```python
from build123d import *

# Parameters (mm, degrees)
SKETCH1_R               = 1.6
BOSS_EXTRUDE1_DEPTH     = 2
SKETCH2_W               = 12
SKETCH2_H               = 12
BOSS_EXTRUDE2_DEPTH     = 6
CUT_EXTRUDE1_DEPTH      = 4
CUT_EXTRUDE1_DEPTH_BACK = 25.093567606
SKETCH2_3_W             = 8
SKETCH2_3_H             = 10
FILLET1_R               = 4
FILLET3_R               = 1
CHAMFER1_SIZE           = 1


with BuildPart() as part:
    # Sketch1 → Boss-Extrude1 (new body)
    with BuildSketch(Plane.XY):
        with BuildLine():
            Line((-12.5, -16.5), (12.5, -16.5))
            ThreePointArc((12.5, -16.5), (15.328427125, -15.328427125), (16.5, -12.5))
            Line((16.5, -12.5), (16.5, 12.5))
            ThreePointArc((16.5, 12.5), (15.328427125, 15.328427125), (12.5, 16.5))
            Line((12.5, 16.5), (-12.5, 16.5))
            ThreePointArc((-12.5, 16.5), (-15.328427125, 15.328427125), (-16.5, 12.5))
            Line((-16.5, 12.5), (-16.5, -12.5))
            ThreePointArc((-16.5, -12.5), (-15.328427125, -15.328427125), (-12.5, -16.5))
        make_face()
        with Locations((-12.5, -12.5)):
            Circle(SKETCH1_R, mode=Mode.SUBTRACT)
        with Locations((12.5, -12.5)):
            Circle(SKETCH1_R, mode=Mode.SUBTRACT)
        with Locations((12.5, 12.5)):
            Circle(SKETCH1_R, mode=Mode.SUBTRACT)
        with Locations((-12.5, 12.5)):
            Circle(SKETCH1_R, mode=Mode.SUBTRACT)
    extrude(amount=BOSS_EXTRUDE1_DEPTH)

    # Sketch2 → Boss-Extrude2 (add)
    with BuildSketch(Plane.XY.offset(2)):
        with Locations((0, -10.5)):
            Rectangle(SKETCH2_W, SKETCH2_H)
    extrude(amount=BOSS_EXTRUDE2_DEPTH)

    # Sketch2<3> → Cut-Extrude1 (cut, two sides: drawn at the far end of the back side and taken through both)
    with BuildSketch(Plane.XY.offset(2).offset(-CUT_EXTRUDE1_DEPTH_BACK)):
        with Locations((0, -11.5)):
            Rectangle(SKETCH2_3_W, SKETCH2_3_H)
    extrude(amount=CUT_EXTRUDE1_DEPTH + CUT_EXTRUDE1_DEPTH_BACK, mode=Mode.SUBTRACT)

    # Fillet1
    fillet1_edges = [part.edges().sort_by_distance(p)[0] for p in [
        (0, -4.5, 8),
    ]]
    fillet(fillet1_edges, radius=FILLET1_R)

    # Fillet3
    fillet3_edges = [part.edges().sort_by_distance(p)[0] for p in [
        (-6, -12.5, 8),
        (-6, -10.5, 2),
        (0, -4.5, 2),
        (6, -10.5, 2),
        (-6, -4.5, 3),
        (6, -4.5, 3),
        (6, -12.5, 8),
        (6, -5.671572875, 6.828427125),
        (-6, -5.671572875, 6.828427125),
    ]]
    fillet(fillet3_edges, radius=FILLET3_R)

    # Chamfer1
    chamfer1_edges = [part.edges().sort_by_distance(p)[0] for p in [
        (-15.328427125, -15.328427125, 2),
        (-9.75, -16.5, 2),
        (15.328427125, -15.328427125, 2),
        (16.5, 0, 2),
        (15.328427125, 15.328427125, 2),
        (0, 16.5, 2),
        (-15.328427125, 15.328427125, 2),
        (-6, -16.5, 5),
        (0, -16.5, 8),
        (9.75, -16.5, 2),
        (6, -16.5, 5),
        (5.707106781, -16.5, 7.707106781),
        (-5.707106781, -16.5, 7.707106781),
        (-16.5, 0, 2),
        (-6.292893219, -16.5, 2.292893219),
        (6.292893219, -16.5, 2.292893219),
    ]]
    chamfer(chamfer1_edges, length=CHAMFER1_SIZE)


solid = part.part
```
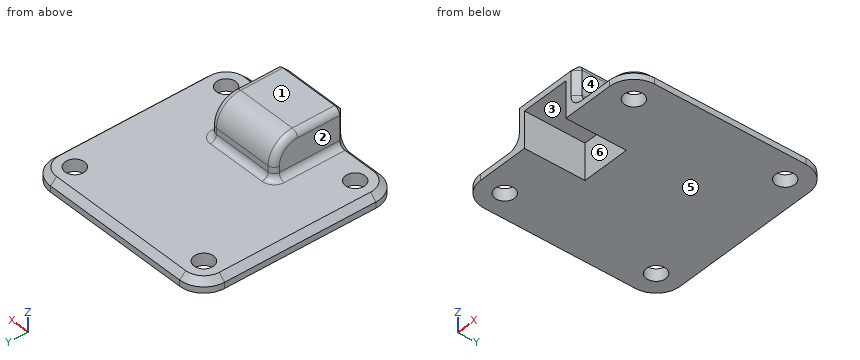
For this review, take the finished solid that the model builds, in its own axes (mm). Face numbers are marked on the shaded views. A direction names the side the tool comes from. Give positions to 0.01 mm unless a question says otherwise; leave off trailing zeros. Write each loop counter-clockwise with the first axis right and the second up, starting at its lowest first coordinate (ties: lowest second). Pieces come first, ordered by that corner, then holes.
Item 1: Take a section at A-A (x = -2). Give the boundary of the cut face in (y, z).
Item 2: The part is to be moulded in two halves that separate along X. For the marked faces 1, 2 and 3, say which applies: +X half, -X half, draft (parallel to the pull), parting line (faces both ways), or undercut.
Item 3: Insertion check: P1, Ø3, axis at y = -12, z = 3, coming from the -X side; P2, Ø4.5, axis at y = -13, z = 5.5, coming from the +X side; P3, Ø3.5, axis at x = -12.5, y = -12.5, coming from the +Z side; P4, Ø1, axis at x = 5.5, y = 5, coming from the -Z side. Each pin has a flat end and moves straight along its axis. Give the tip position at first contact, or say it passes through.
Item 4: Machinability: for the marked faces 4, 5 and 6, which of the approach directions +Z, -Z, +X, -X, +Y, -Y give a long, thin tool a straight path to every point of the face, cutting with its end or side? Answer none if there is none.
Item 5: Wall thickness on probe 1 along Z at (x, y) = (15.5, -11.5); probe 2 along X at (y, z) = (-13.5, 5); probe 3 along Z at (x, y) = (-2.5, -9): over which ranges is each line inside the solid? List them lowest first.
Item 6: Take a section at B-B (y = -10.5). Give the boundary of the cut face in (x, z), and give its area (3 significant figures).
Item 7: Take a section at C-C (y = 7.5). Give the boundary of the cut face in (x, z).
Established:
1. outline: (-16.5, 6) - (-6.5, 6) - (-6.5, 0) - (16.5, 0) - (16.5, 1) - (15.5, 2) - (-3.5, 2) arc R1 cw to (-4.5, 3) - (-4.5, 4) arc R4 ccw to (-8.5, 8) - (-15.5, 8) - (-16.5, 7) - close
2. face 1: draft
2. face 2: -X half
2. face 3: undercut
3. P1: stops at x = -16
3. P2: stops at x = 6
3. P3: stops at z = 2
3. P4: stops at z = 0
4. face 4: +Z, +X, +Y, -Y
4. face 5: -Z, +X, -X, +Y, -Y
4. face 6: -Z, -Y
5. probe 1: z = 0 to 2
5. probe 2: x = -6 to -4, 4 to 6
5. probe 3: z = 6 to 8
6. outline: (-16.5, 0) - (-4, 0) - (-4, 6) - (4, 6) - (4, 0) - (16.5, 0) - (16.5, 1) - (15.5, 2) - (7, 2) arc R1 cw to (6, 3) - (6, 7) arc R1 ccw to (5, 8) - (-5, 8) arc R1 ccw to (-6, 7) - (-6, 3) arc R1 cw to (-7, 2) - (-15.5, 2) - (-16.5, 1) - close
6. area: 89.0 mm2
7. outline: (-16.5, 0) - (16.5, 0) - (16.5, 1) - (15.5, 2) - (-15.5, 2) - (-16.5, 1) - close
